Here's how the part is built. I have some questions about the finished solid (model axes, mm). A direction names the side the tool comes from. Give positions to 0.01 mm unless a question says otherwise; leave off trailing zeros. Order: outer loops, then holes, each group sorted by start corner. A loop starts at its lowest first (then second) coordinate and runs counter-clockwise, first axis right, second up.
Autodesk Inventor part; units mm, degrees
ref_plane "Plan de courroie" through (0, 19.65, 11) normal (0, 0, 1) x (1, 0, 0)
ref_plane "YZ Plane" through (0, 0, 0) normal (1, 0, 0) x (0, 1, 0)
ref_plane "XZ Plane" through (0, 0, 0) normal (0, 1, 0) x (-1, 0, 0)
sketch "Esquisse principale" plane through (0, 0, 0) normal (1, 0, 0) x (0, 1, 0)
  line L0 (0, 22) -> (30.65, 22)
  line L1 (30.65, 22) -> (30.65, 18.6115)
  line L2 (30.65, 18.6115) -> (19.65, 15.2484)
  line L3 (19.65, 15.2484) -> (19.65, 6.7516)
  line L4 (19.65, 6.7516) -> (30.65, 3.3885)
  line L5 (30.65, 3.3885) -> (30.65, 0)
  line L6 (30.65, 0) -> (0, 0)
  line L7 (28.65, 18) -> (28.65, 4) construction
  line L8 (19.65, 11) -> (28.65, 11) construction
  line L9 (30.65, 18.6115) -> (30.65, 3.3885)
  line L10 (0, -4.4) -> (0, 26.4)
  line L11 (0, 0) -> (0, 22)
  dimension "d0" = 14
  dimension "d1" = 34
  dimension "d2" = 2
  dimension "d6" = 22
  dimension "d21" = 57.3
  dimension "d25" = 11
  dimension "d27" = 11
ref_plane "Plan de courroie" through (0, 19.65, 11) normal (0, 0, 1) x (1, 0, 0)
revolve "Corps" add sketch "Esquisse principale" angle 360 about axis through (0, 0, -10) along (0, 0, 1)
revolve "Bord" cut sketch "Esquisse principale" angle 360 about axis through (0, 0, -10) along (0, 0, 1) contours L9 L4 L3 L2
fillet "Congé externe" [suppressed]
fillet "Congé interne" [suppressed]
pattern_of_one "Réseau de bords"
sketch "Esquisse5" plane through (0, 0, 0) normal (1, 0, 0) x (0, 1, 0)
  line L0 (0, -3.4128) -> (0, 36.612)
  line L1 (-30.65, 22) -> (30.65, 22)
  line L2 (0, 22.15) -> (17.6, 22.15)
  line L3 (0, -0.15) -> (16, -0.15)
  line L4 (16, -0.15) -> (17.6, 22.15)
  line L5 (-30.65, 0) -> (30.65, 0)
  point P0 (0, 0)
  point P1 (0, 0)
  point P2 (16.0108, 0)
  point P3 (17.5892, 22)
  point P4 (0, 22)
  dimension "d42" = 17.6
  dimension "d43" = 16
  dimension "d44" = 22.3
  dimension "d45" = 0.15
revolve "Révolution4" cut sketch "Esquisse5" angle 360 about axis through (0, 0, -3.4128) along (0, 0, 1) contours L0 L1 L4 L5
sketch "Esquisse6" plane through (0, 0, 22) normal (0, 0, 1) x (1, 0, 0)
  circle A0 centre (0, 0) radius 16.865
  line L0 (0, 0) -> (0, -20.3101)
  line L1 (0, 0) -> (20.7504, 0)
  line L2 (0, 0) -> (-20.5452, 0)
  point P0 (0, -16.865)
  point P1 (-16.865, 0)
  point P2 (16.865, 0)
  dimension "d54" = 33.73
hole "Perçage2" at (0, -16.865, 22) at (-16.865, 0, 22) at (16.865, 0, 22) direction (0, 0, -1) diameter 5.1881 depth 15 tip angle 118
equation "\"d0\" = da_Bw"
equation "\"d1\" = da_Alfa"
equation "\"d2\" = da_c"
equation "\"d21\" = da_Dw"
equation "\"d25\" = da_Hd"
equation "\"d27\" = da_Se"
equation "\"da_r1\" = 0"
equation "\"da_r2\" = 0"
equation "\"d18\" = da_Sg"
equation "\"d5\" = da_Se"
equation "\"da_Bw\" = 14"
equation "\"da_Alfa\" = 34deg"
equation "\"da_c\" = 2"
equation "\"da_Dw\" = 57.3"
equation "\"da_Hd\" = 11"
equation "\"da_Se\" = 11"
equation "\"da_Sg\" = 12"
properties part number "Poulie à gorge2" material "Steel"
Q1. I'm going to push flat-ended pins straight in: P1, Ø3, axis at x = 2.5, z = 12.5, coming from the +Y side; P2, Ø4, axis at x = 0, y = -16.865, coming from the -Z side; P3, Ø3, axis at x = -16.865, y = 0, coming from the +Z side; P4, Ø8, axis at y = -8.5, z = 17.5, coming from the -X side. Where does each tip first touch, or does it pass through?
Filled sheet:
P1: stops at y = 19.62
P2: stops at z = 0
P3: stops at z = 6.34
P4: stops at x = -30.29
Q2. If we section it at A-A on z = 2: List the corners of the cut face in (x, y) for me, plus the area to 3 significant figures.
Filled sheet:
outline: circle Ø61.3 at (0, 0); hole circle Ø32.31 at (0, 0)
area: 2,130 mm2
Q3. Thinking about a two-plate mould opening in X: for faces 1 (the face through (-6.11, 19.4, 15.46)), 2 (the face through (13, 13, 22)), 3 (the face through (-17.6, 0.2, 5.9)), 4 (the face through (19.46, 0.06, 14.39)), which applies, released by +X, released by -X, zero draft, split by the parting line, or undercut?
Filled sheet:
face 1: split by the parting line
face 2: zero draft
face 3: undercut
face 4: undercut
Q4. I need wall thicknesses on L1, parallel to X at y = 0, z = 12; L2, parallel to Y at x = -5.5, z = 3; L3, parallel to X at y = -15, z = 11. Which ranges of each line are inside material? Lowest first, please.
Filled sheet:
L1: x = -19.65 to -19.46, 19.46 to 19.65
L2: y = -30.15 to -15.27, 15.27 to 30.15
L3: x = -12.69 to -7.57, 7.57 to 12.69
Q5. For faces 5 (the face through (0.06, -19.46, 14.39)), 6 (the face through (-19.854, -4.409, 6.541)), 7 (the face through (25.844, 16.477, 20.282)), which set-ups out of +Z, -Z, +X, -X, +Y, -Y let a thin tool reach every point of the face, with its end or its side?
Filled sheet:
face 5: +Z
face 6: none
face 7: +Z, -Z
